Model file for the job. Use its own axes, mm. Face numbers are marked on the shaded views. A direction names the side the tool comes from. Give positions to 0.01 mm unless a question says otherwise; leave off trailing zeros. Write each loop counter-clockwise with the first axis right and the second up, starting at its lowest first coordinate (ties: lowest second). Pieces come first, ordered by that corner, then holes. Notation, with made-up numbers: M 0,54.25 L 52,54.25 A20 ccw 52,69.25 Z; hole C -39.5,57.25 d7. An arc over 180 degrees is marked long. Answer as a JSON object with one key per item and string values. Group by question number.
```python
from build123d import *

# Parameters (mm, degrees)
BASE_FLANGE1_DEPTH  = 2
SKETCH6_R           = 1
CUT_EXTRUDE1_DEPTH  = 0.5
SKETCH8_R           = 0.45
BOSS_EXTRUDE1_DEPTH = 1


# Sheet-metal steps are written as plain solids
with BuildPart() as part:
    # Sketch1 → Base-Flange1 (new body)
    with BuildSketch(Plane.XY):
        with BuildLine():
            Line((10.5, -2), (0, -2))
            ThreePointArc((0, -2), (-2, 0), (0, 2))
            Line((0, 2), (10.5, 2))
            ThreePointArc((10.5, 2), (12.5, 0), (10.5, -2))
        make_face()
    extrude(amount=-BASE_FLANGE1_DEPTH)

    # Sketch6 → Cut-Extrude1 (cut)
    with BuildSketch(Plane.XY):
        Circle(SKETCH6_R)
        with Locations((10.5, 0)):
            Circle(SKETCH6_R)
    extrude(amount=-CUT_EXTRUDE1_DEPTH, mode=Mode.SUBTRACT)

    # Sketch8 → Boss-Extrude1 (add)
    with BuildSketch(Plane.XY):
        with Locations((4, 0)):
            Circle(SKETCH8_R)
        with Locations((6.5, 0)):
            Circle(SKETCH8_R)
    extrude(amount=BOSS_EXTRUDE1_DEPTH)


solid = part.part
```
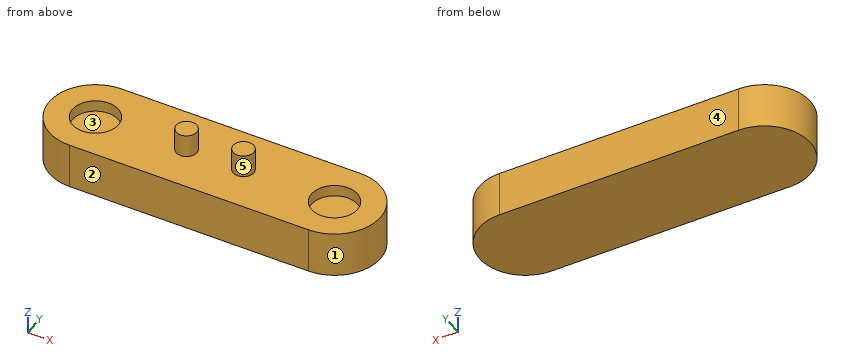
Q1. Drop a flat-ended pin along its axis: P1, Ø1.6, axis at x = 10.5, y = 0.5, coming from the +Z side. Give the stop position or say it passes through.
Q2. 3-axis set-ups, long thin cutter, end or side, ignore diameter. For the marked faces 4 and 5: which of +Z, -Z, +X, -X, +Y, -Y reach the whole face in a straight line?
Q3. Slice it at B-B, the plane x = 4.25. Write the cut outline in (y, z), then the cut area to 3 significant figures.
Q4. Slice it at A-A, the plane y = 0. Write the cut outline in (x, z).
Q5. Slice it at D-D, the plane y = 1.2. Write the cut outline in (x, z).
Q6. Two-plate mould, pull along Y, no slides. Class the marked faces 1, 2 and 3: +Y half, -Y half, draft (parallel to the pull), parting line (faces both ways), or undercut.
Q7. Slice it at C-C, the plane z = -0.7. Write the cut outline in (x, y), then the cut area to 3 significant figures.
Q8. Wall check: L1, parallel to Y at x = 0, z = -0.4; L2, parallel to Z at x = 6, y = 1.75; L3, parallel to Z at x = 0.75, y = -0.1. Give the ranges that are in metal, low to high.
Solved:
{
 "1": {"P1": "stops at z = 0"},
 "2": {"face 4": "+Z, -Z, +X, -X, +Y", "face 5": "+Z"},
 "3": {"outline": "M -2,-2 L 2,-2 L 2,0 L 0.37,0 L 0.37,1 L -0.37,1 L -0.37,0 L -2,0 Z", "area": "8.75 mm²"},
 "4": {"outline": "M -2,-2 L 12.5,-2 L 12.5,0 L 11.5,0 L 11.5,-0.5 L 9.5,-0.5 L 9.5,0 L 6.95,0 L 6.95,1 L 6.05,1 L 6.05,0 L 4.45,0 L 4.45,1 L 3.55,1 L 3.55,0 L 1,0 L 1,-0.5 L -1,-0.5 L -1,0 L -2,0 Z"},
 "5": {"outline": "M -1.6,-2 L 12.1,-2 L 12.1,0 L -1.6,0 Z"},
 "6": {"face 1": "parting line", "face 2": "-Y half", "face 3": "undercut"},
 "7": {"outline": "M 0,-2 L 10.5,-2 A2 ccw 10.5,2 L 0,2 A2 ccw Z", "area": "54.6 mm²"},
 "8": {"L1": "y = -2 to -1, 1 to 2", "L2": "z = -2 to 0", "L3": "z = -2 to -0.5"}
}
